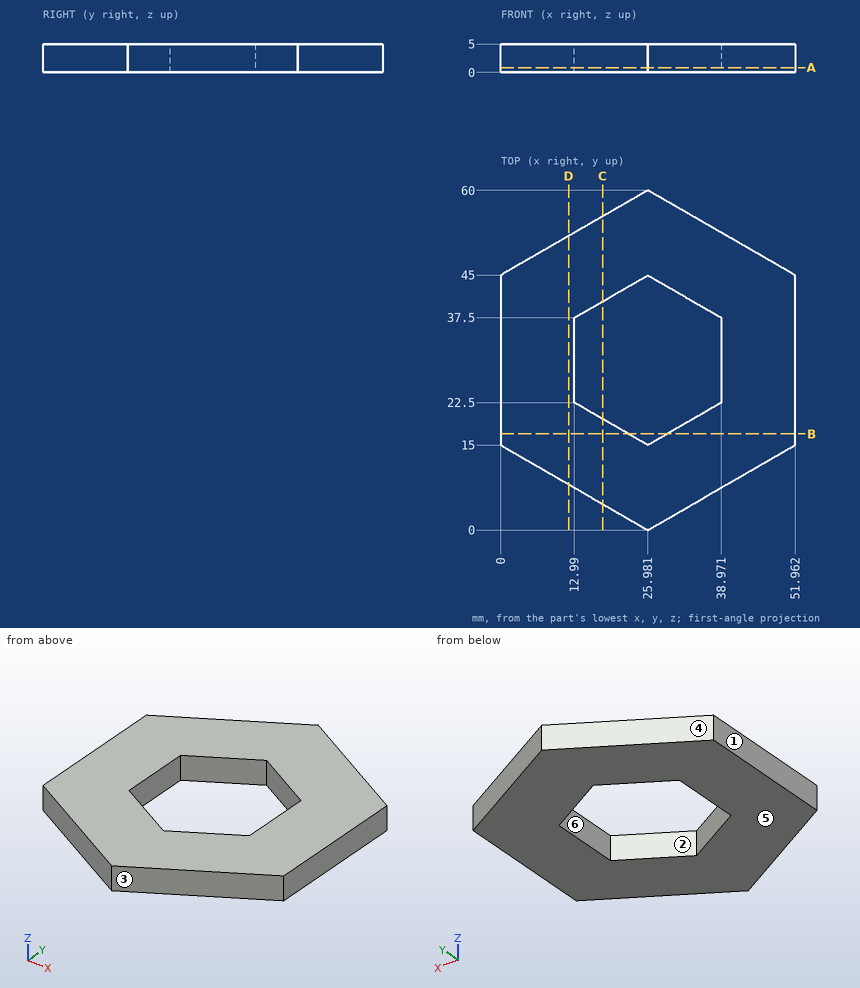
Here's the drawing with two shaded views (mm, measured from the low corner). I have some questions. A direction names the side the tool comes from. Round coordinates to 2 decimals unless told otherwise and drop trailing zeros. Loops run counter-clockwise (first coordinate to the right, second up) from the corner with the lowest first, then second, coordinate; pieces in that order, holes last. Notation, with made-up numbers: M 36,23.25 L 70,23.25 A23 cw 70,48.25 Z; hole C 38.5,-6 d2. An arc over 180 degrees is marked long. Answer as a JSON object with one key per item and string values. Group by question number.
Q1. Imagine slicing it at A-A, the plane z = 0.85. Please give me the cut outline in (x, y), then the cut area to 3 significant figures.
Q2. Imagine slicing it at C-C, the plane x = 18. Please give me the cut outline in (y, z), then the cut area to 3 significant figures.
Q3. We'd pull the mould along Y, two halves only. Please class the marked faces 1, 2, 3 and 4: +Y half, -Y half, draft (parallel to the pull), parting line (faces both ways), or undercut.
Q4. Please list where these lines run through material, in increasing order: L1, parallel to X at y = 36.5, z = 1.75; L2, parallel to X at y = 38, z = 0.55 (1 decimal); L3, parallel to Y at x = 34.5, z = 1.45.
Q5. Imagine slicing it at D-D, the plane x = 12. Please give me the cut outline in (y, z).
Q6. Will this pin go through, and if not, where does the flat tip stop? pin 1 (2 mm diameter, centred on y = 53.5, z = 1.5, fed in from +X).
Q7. On a 3-axis mill with a long thin cutter (end or side, diameter ignored), from which of +Z, -Z, +X, -X, +Y, -Y can I reach the whole of each face in a straight line? I mean the marked faces 5 and 6. Say none if no direction works.
Q8. Imagine slicing it at B-B, the plane y = 17. Please give me the cut outline in (x, z) (1 decimal), then the cut area to 3 significant figures.
Findings:
{
 "1": {"outline": "M 0,15 L 25.98,0 L 51.96,15 L 51.96,45 L 25.98,60 L 0,45 Z; hole M 12.99,22.5 L 25.98,15 L 38.97,22.5 L 38.97,37.5 L 25.98,45 L 12.99,37.5 Z", "area": "1,750 mm2"},
 "2": {"outline": "M 4.61,0 L 19.61,0 L 19.61,5 L 4.61,5 Z; M 40.39,0 L 55.39,0 L 55.39,5 L 40.39,5 Z", "area": "150 mm2"},
 "3": {"face 1": "draft", "face 2": "undercut", "face 3": "-Y half", "face 4": "+Y half"},
 "4": {"L1": "x = 0 to 12.99, 38.97 to 51.96", "L2": "x = 0 to 13.9, 38.1 to 52", "L3": "y = 4.92 to 19.92, 40.08 to 55.08"},
 "5": {"outline": "M 8.07,0 L 51.93,0 L 51.93,5 L 8.07,5 Z"},
 "6": {"pin 1": "stops at x = 38.97"},
 "7": {"face 5": "-Z, +X, -X, +Y, -Y", "face 6": "+Z, -Z"},
 "8": {"outline": "M 0,0 L 22.5,0 L 22.5,5 L 0,5 Z; M 29.4,0 L 52,0 L 52,5 L 29.4,5 Z", "area": "225 mm2"}
}
